For this review, take the finished solid that the model builds, in its own axes (mm). A direction names the side the tool comes from. Give positions to 0.01 mm unless a question says otherwise; leave off trailing zeros. Write each loop counter-clockwise with the first axis right and the second up, starting at its lowest first coordinate (ties: lowest second). Pieces come first, ordered by that corner, then holes. Notation, with made-up numbers: M -34.75,34.5 L 2.25,34.5 A16 ccw 2.25,46.5 Z; hole C 66.5,79.25 d5. An arc over 180 degrees is marked long. One line per item, written item: value. Start each with the question number.
Item 1: Tool access review of faces 4 (the face through (-4.36, 4.12, 3.24)), 5 (the face through (4.5, 2.5, 1.5)), 6 (the face through (-6.972, -1.924, 1.268)): name each direction out of +Z, -Z, +X, -X, +Y, -Y from which nothing blocks a thin tool from reaching the whole face with its end or side.
Item 2: Consider section A-A, the plane x = 14. Write out the cut boundary in (y, z), and give its area (3 significant figures).
Item 3: Consider section B-B, the plane z = 1.05. Write out the cut boundary in (x, y).
Item 4: Mouldability with a two-part tool opening along Y and no side actions: class faces 1 (the face through (-2, 2, 6)), 2 (the face through (-3, 2.5, 1.5)), 3 (the face through (-4.85, 6.36, 1.23)) as released by +Y, released by -Y, zero draft, split by the parting line, or undercut.
Item 5: Consider section C-C, the plane y = -1. Write out the cut boundary in (x, z).
Item 6: Clearance check with flat-ended pins moving along their axes: pin 1 Ø2 at (y, z) = (-2, 1.5) entering from -X; pin 2 Ø0.6 at (y, z) = (-7, 2) entering from -X; pin 3 Ø1.2 at (x, z) = (2, 1) entering from -Y. State where each tip first meets the part, or that it passes through.
Item 7: Consider section D-D, the plane x = 0. Write out the cut boundary in (y, z).
Item 8: To check wall thickness, follow probe 1 along Y at (x, z) = (14, 1.8); probe 2 along Y at (x, z) = (-3, 0.5); probe 3 along X at (y, z) = (2.5, 0.45). State the ranges of each line that lie inside material, in increasing order.
Autodesk Inventor part; units mm, degrees
ref_plane "YZ Plane" through (0, 0, 0) normal (1, 0, 0) x (0, 1, 0)
ref_plane "XZ Plane" through (0, 0, 0) normal (0, 1, 0) x (-1, 0, 0)
ref_plane "XY Plane" through (0, 0, 0) normal (0, 0, 1) x (1, 0, 0)
sketch "MCP joint" plane through (0, 0, 0) normal (0, 0, 1) x (1, 0, 0)
  point P0 (0, 0)
  point P1 (0, 0)
sketch "Sketch2" plane through (0, 0, 0) normal (0, 0, 1) x (1, 0, 0)
  line L0 (9, -7.5) -> (16, -7.5)
  line L1 (16, -7.5) -> (16, 10.5)
  line L2 (16, 10.5) -> (9, 10.5)
  circle A0 centre (0, 0) radius 8
  line L3 (9, 10.5) -> (-1.9428, 7.7605)
  line L4 (9, -7.5) -> (0.4552, -7.987)
  point P0 (16, 1.5)
  point P1 (3.5, 1.5)
  point P2 (16, 1.5)
  dimension "d0" = 18
  dimension "d3" = 16
  dimension "d94" = 1.5
  dimension "d95" = 16
  dimension "d96" = 9
  dimension "d97" = 9
extrude "base" add sketch "Sketch2" along normal blind 2.5
sketch "Sketch3" plane through (0, 0, 2.5) normal (0, 0, 1) x (1, 0, 0)
  point P0 (0, 0)
  point P1 (0, 0)
hole "bearing pocket" at (0, 0, 2.5) direction (0, 0, -1) diameter 4 end through all
sketch "Sketch13" plane through (0, 0, 0) normal (0, 0, -1) x (-1, 0, 0)
  line L0 (-9, -7.5) -> (-9, -5)
  arc A0 (-0.4552, -7.987) -> (1.9428, 7.7605) centre (0, 0) ccw
  line L1 (-9, -5) -> (6.245, -5)
  line L2 (-0.4552, -7.987) -> (-9, -7.5)
  dimension "d76" = 2.5
extrude "bottom cutout" cut sketch "Sketch13" against normal through all
fillet "Fillet2" radius 2 1 edges at (9, -5, 1.25)
fillet "Fillet4" radius 6 1 edges at (-6.245, -5, 1.25)
sketch "Sketch7" plane through (0, 0, 0) normal (0, 0, -1) x (-1, 0, 0)
  line L0 (3, 2.5) -> (-4.5, 2.5) construction
  line L1 (-4.5, 2.5) -> (-4.5, -2.5) construction
  line L2 (-4.5, -2.5) -> (3, -2.5) construction
  line L3 (3, -2.5) -> (3, 2.5) construction
  line L4 (3, 2.5) -> (-4.5, -2.5) construction
  line L5 (-4.5, 2.5) -> (3, -2.5) construction
  point P0 (0, 0)
  point P1 (-0.75, 0)
  point P2 (0, 0)
  point P3 (-0.75, 0)
  dimension "d34" = 3
  dimension "d35" = 4.5
  dimension "d36" = 5
hole "potentiometer pins" at (-3, 2.5, 0) at (-3, -2.5, 0) at (4.5, -2.5, 0) at (4.5, 2.5, 0) direction (0, 0, 1) diameter 1 depth 1.5
sketch "Sketch8" plane through (0, 0, 2.5) normal (0, 0, 1) x (1, 0, 0)
  line L0 (8.1428, 0) -> (0, 0) construction
  line L1 (0, 0) -> (-8.8782, 8.8782) construction
  circle A0 centre (-1.4142, 1.4142) radius 3.5
  dimension "d45" = 2
  dimension "d46" = 7
  dimension "d59" = 45
extrude "bearing" add sketch "Sketch8" along normal blind 3.5
sketch "Sketch10" plane through (0, 0, 2.5) normal (0, 0, 1) x (1, 0, 0)
  circle A0 centre (-1.4142, 1.4142) radius 3.5
  circle A1 centre (-1.4142, 1.4142) radius 4
  point P0 (0, 0)
  point P1 (1.0607, -1.0607)
  dimension "d56" = 8
extrude "bearing spacer" add sketch "Sketch10" along normal blind 1.5
sketch "Sketch11" plane through (-1.4142, 1.4142, 6) normal (0, 0, 1) x (1, 0, 0)
  point P0 (1.4142, -1.4142)
  point P1 (1.4142, -1.4142)
hole "Hole4" at (0, 0, 6) direction (0, 0, -1) diameter 4.2 end through all
sketch "Sketch12" plane through (0, 0, 2.5) normal (0, 0, 1) x (1, 0, 0)
  point P0 (0, 0)
  point P1 (14, 4)
  point P2 (14, -1)
  point P3 (0, 0)
  dimension "d88" = 14
  dimension "d89" = 14
  dimension "d90" = 4
  dimension "d91" = 1
hole "mounting" at (14, 4, 2.5) at (14, -1, 2.5) direction (0, 0, -1) diameter 2.4 end through all
equation "\"MCP_spring_arm\" = F5_MCP_spring_arm"
properties part number "MCP mount M F5"
Model answer:
1. face 4: +Z
1. face 5: -Z
1. face 6: +Z, -Z, -X
2. outline: M -7.5,0 L -2.2,0 L -2.2,2.5 L -7.5,2.5 Z; M 0.2,0 L 2.8,0 L 2.8,2.5 L 0.2,2.5 Z; M 5.2,0 L 10.5,0 L 10.5,2.5 L 5.2,2.5 Z
2. area: 33.0 mm2
3. outline: M -6.93,4 A6 ccw -1.73,-5 L 7,-5 A2 cw 9,-7 L 9,-7.5 L 16,-7.5 L 16,10.5 L 9,10.5 L -1.94,7.76 A8 ccw Z; hole C -3,-2.5 d1; hole C -3,2.5 d1; hole C 0,0 d4.2; hole C 4.5,-2.5 d1; hole C 4.5,2.5 d1; hole C 14,-1 d2.4; hole C 14,4 d2.4
4. face 1: zero draft
4. face 2: undercut
4. face 3: released by +Y
5. outline: M -7.39,0 L -1.85,0 L -1.85,6 L -3.95,6 L -3.95,4 L -4.6,4 L -4.6,2.5 L -7.39,2.5 Z; M 1.85,0 L 12.8,0 L 12.8,2.5 L 1.85,2.5 Z; M 15.2,0 L 16,0 L 16,2.5 L 15.2,2.5 Z
6. pin 1: stops at x = -7.39
6. pin 2: stops at x = 8.98
6. pin 3: stops at y = -5
7. outline: M -5,0 L -2.1,0 L -2.1,4 L -2.33,4 L -2.33,2.5 L -5,2.5 Z; M 2.1,0 L 8.25,0 L 8.25,2.5 L 5.16,2.5 L 5.16,4 L 4.62,4 L 4.62,6 L 2.1,6 Z
8. probe 1: y = -7.5 to -2.2, 0.2 to 2.8, 5.2 to 10.5
8. probe 2: y = -4.86 to -3, -2 to 2, 3 to 7.42
8. probe 3: x = -7.54 to -3.5, -2.5 to 4, 5 to 16
